Could you check a few things on this model? Use its own coordinates, in mm. Face numbers are marked on the shaded views. A direction names the side the tool comes from. Give positions to 0.01 mm unless a question says otherwise; leave off trailing zeros. Loops run counter-clockwise (first coordinate to the right, second up) from the corner with the lowest first, then second, coordinate; pieces in that order, holes last. Notation, with made-up numbers: (-35.5, 31) -> (-11.5, 31) arc R14 ccw to (-11.5, 40) -> close; hole circle Ø6 at (-21, -31.75). An arc over 180 degrees is marked (long way). Write each question's results on one line, items separated by ' | '. Start each with the question number.
Q1. Will these pins go through, and if not, where does the flat tip stop? P1, Ø8, axis at y = -70.5, z = 21, coming from the +X side; P2, Ø1.5, axis at y = -41.5, z = 44.5, coming from the +X side; P3, Ø10, axis at x = 55, y = -67.5, coming from the +Z side.
Q2. If we section it at B-B, the plane z = 30.5: List the corners of the cut face in (x, y) for me.
Q3. We'd pull the mould along X, two halves only. Please class the marked faces 1, 2 and 3: released by +X, released by -X, zero draft, split by the parting line, or undercut.
Q4. If we section it at D-D, the plane y = -44.5: List the corners of the cut face in (x, z) for me, plus the area to 3 significant figures.
Q5. If I drill on line 1 along X through (y, z) = (-19.5, 34); line 2 along Z through (x, y) = (10.5, -40.5); line 3 along X through (y, z) = (-37.5, 55), over which ranges is the centre line in solid material (lowest first)?
Q6. If we section it at C-C, the plane x = 22.5: List the corners of the cut face in (y, z) for me, plus the area to 3 significant figures.
Q7. Which directions (+Z, -Z, +X, -X, +Y, -Y) give clear straight access to the entire face, cutting with the end or side of a thin tool? Please do the marked faces 4, 5 and 6.
Q8. If we section it at A-A, the plane y = -104: List the corners of the cut face in (x, z) for me, plus the area to 3 significant figures.
from build123d import *

# Parameters (mm, degrees)
F0_W     = 152.4
F0_H     = 127
F1_DEPTH = 127
F3_DEPTH = 76.2
F4_W     = 38.972323
F4_H     = 43.56414
F5_DEPTH = 50.801
F6_R     = 17.360995
F7_DEPTH = 58.177971
F8_SIZE  = 25.4
F9_R     = 50.8


with BuildPart() as f1:
    # F0 (on Front) → F1 (new body)
    with BuildSketch(Plane.XZ):
        with Locations((1.744647, 5.323029)):
            Rectangle(F0_W, F0_H)
    extrude(amount=F1_DEPTH)

    # F2 (on face) → F3 (cut)
    with BuildSketch(Plane.XZ.offset(127)):
        Polygon((1.744647, 68.823029), (0, 68.823029), (0, 0), (77.944647, 0), (77.944647, 68.823029), align=None)
    extrude(amount=-F3_DEPTH, mode=Mode.SUBTRACT)

    # F4 (on face) → F5 (cut, through all)
    with BuildSketch(Plane.XZ.offset(50.8)):
        with Locations((19.486161, 47.040959)):
            Rectangle(F4_W, F4_H)
    extrude(amount=-F5_DEPTH, mode=Mode.SUBTRACT)

    # F6 (on face) → F7 (cut, through all)
    with BuildSketch(Plane.XY):
        with Locations((36.480688, -90.639494)):
            Circle(F6_R)
    extrude(amount=-F7_DEPTH, mode=Mode.SUBTRACT)

    # F8
    f8_edges = [f1.edges().sort_by_distance(p)[0] for p in [
        (77.944647, -25.4, 68.823029),
    ]]
    chamfer(f8_edges, length=F8_SIZE)

    # F9
    f9_edges = [f1.edges().sort_by_distance(p)[0] for p in [
        (-37.227677, -127, 68.823029),
    ]]
    fillet(f9_edges, radius=F9_R)


solid = f1.part
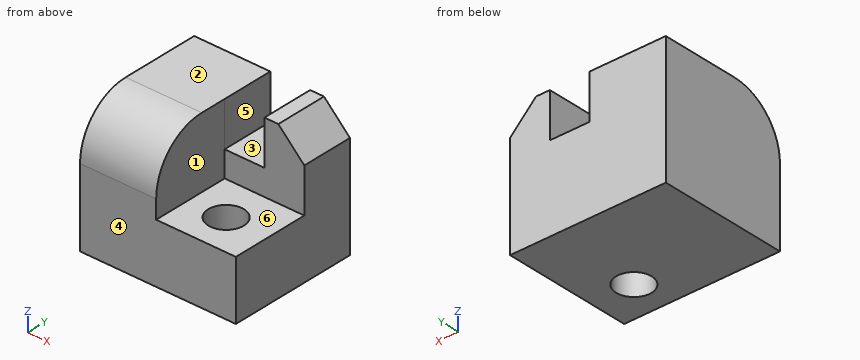
Final values:
1) P1: stops at x = 0 | P2: stops at x = 77.62 | P3: stops at z = 0
2) outline: (-74.46, -125.44) -> (0, -125.44) -> (0, 0) -> (-74.46, 0) -> close; (38.97, -50.8) -> (77.94, -50.8) -> (77.94, 0) -> (38.97, 0) -> close
3) face 1: released by +X | face 2: zero draft | face 3: undercut
4) outline: (-74.46, -58.18) -> (77.94, -58.18) -> (77.94, 43.42) -> (52.54, 68.82) -> (38.97, 68.82) -> (38.97, 25.26) -> (0, 25.26) -> (0, 68.82) -> (-74.46, 68.82) -> close | area: 17,300 mm²
5) line 1: x = -74.46 to 0, 38.97 to 77.94 | line 2: z = -58.18 to 25.26 | line 3: x = -74.46 to 0, 38.97 to 66.37
6) outline: (-127, -58.18) -> (-100.93, -58.18) -> (-100.93, 0) -> (-127, 0) -> close; (-80.35, -58.18) -> (0, -58.18) -> (0, 25.26) -> (-50.8, 25.26) -> (-50.8, 0) -> (-80.35, 0) -> close | area: 7,470 mm²
7) face 4: +Z, -Z, +X, -X, -Y | face 5: +Z, +Y, -Y | face 6: +Z, +X, -Y
8) outline: (-74.46, -58.18) -> (25.39, -58.18) -> (25.39, 0) -> (0, 0) -> (0, 60.54) -> (-74.46, 60.54) -> close; (47.57, -58.18) -> (77.94, -58.18) -> (77.94, 0) -> (47.57, 0) -> close | area: 12,100 mm²
